Geometry check sheet. Reference: drawing and pictorial views, mm from the part's lowest x, y, z. A direction names the side the tool comes from. Coordinates: 2 decimals unless noted, no trailing zeros. Loops run counter-clockwise (first coordinate to the right, second up) from the corner with the lowest first, then second, coordinate; pieces in that order, holes last. Notation, with made-up numbers: (-31.75, 49) -> (17.25, 49) arc R12 cw to (17.25, 57) -> close; hole circle Ø1 at (51, -21.75). An arc over 180 degrees is marked (long way). Use one line per item in the form item = value.
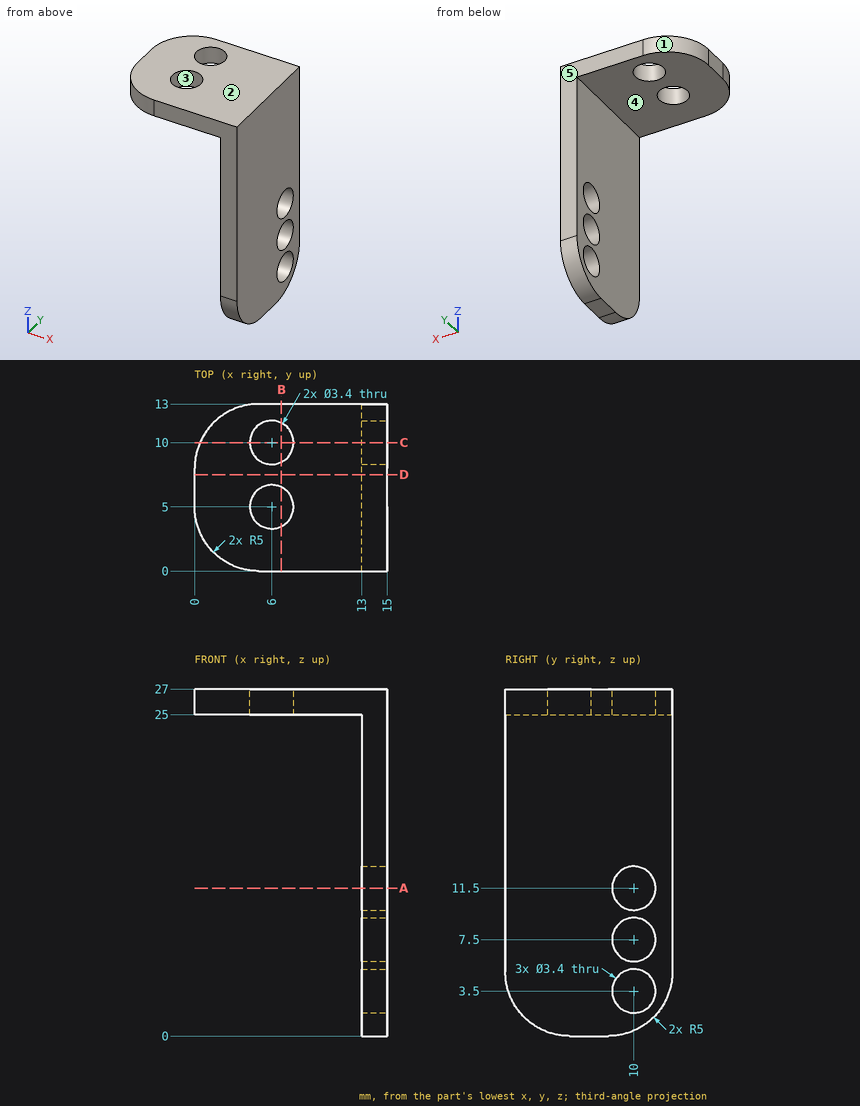
(1) Mould release check, pull along X, two halves, no side actions. Record for the marked faces 1, 2 and 3: +X half, -X half, draft (parallel to the pull), parting line (faces both ways), or undercut.
Established:
face_1 = -X half
face_2 = draft
face_3 = undercut
(2) Tool access check on the marked faces 4 and 5. Record the directions out of +Z, -Z, +X, -X, +Y, -Y that give a thin tool (end or side, any length) a straight path to the whole face; none if there is none.
Established:
face_4 = -Z, -X, +Y, -Y
face_5 = +Z, -Z, +X, -X, +Y
(3) Section check D-D, the plane y = 7.5. Record the boundary of the cut face in (x, z).
Established:
outline = (0, 25) -> (13, 25) -> (13, 0) -> (15, 0) -> (15, 27) -> (0, 27) -> close
(4) Section check A-A, the plane z = 11.5. Record the boundary of the cut face in (x, y), plus the area to 3 significant figures.
Established:
outline = (13, 0) -> (15, 0) -> (15, 8.3) -> (13, 8.3) -> close; (13, 11.7) -> (15, 11.7) -> (15, 13) -> (13, 13) -> close
area = 19.2 mm²
(5) Section check B-B, the plane x = 6.75. Record the boundary of the cut face in (y, z), plus the area to 3 significant figures.
Established:
outline = (0, 25) -> (3.47, 25) -> (3.47, 27) -> (0, 27) -> close; (6.53, 25) -> (8.47, 25) -> (8.47, 27) -> (6.53, 27) -> close; (11.53, 25) -> (13, 25) -> (13, 27) -> (11.53, 27) -> close
area = 13.8 mm²
(6) Section check C-C, the plane y = 10. Record the boundary of the cut face in (x, z), plus the area to 3 significant figures.
Established:
outline = (0.42, 25) -> (4.3, 25) -> (4.3, 27) -> (0.42, 27) -> close; (7.7, 25) -> (13, 25) -> (13, 13.2) -> (15, 13.2) -> (15, 27) -> (7.7, 27) -> close; (13, 0.42) -> (15, 0.42) -> (15, 1.8) -> (13, 1.8) -> close; (13, 5.2) -> (15, 5.2) -> (15, 5.8) -> (13, 5.8) -> close; (13, 9.2) -> (15, 9.2) -> (15, 9.8) -> (13, 9.8) -> close
area = 51.1 mm²
(7) Go/stop test with flat-tipped pins: P1, Ø2.5, axis at x = 6, y = 5, coming from the +Z side; P2, Ø4.5, axis at y = 10, z = 3.5, coming from the -X side; P3, Ø3, axis at x = 2, y = 10.5, coming from the -Z side. Record where each tip stops, or that it passes through.
Established:
P1 = through
P2 = 13
P3 = 25
(8) Scan lines: line 1 along Y through (x, z) = (6, 25.5); line 2 along Z through (x, y) = (13.6, 10); line 3 along Z through (x, y) = (6, 1.5). Record each from-to range of solid material in increasing order.
Established:
line_1 = 0 to 3.3, 6.7 to 8.3, 11.7 to 13
line_2 = 0.42 to 1.8, 5.2 to 5.8, 9.2 to 9.8, 13.2 to 27
line_3 = 25 to 27
